Build history of the part. All positions in model axes, mm. Round coordinates to 2 decimals unless told otherwise and drop trailing zeros. Write each loop counter-clockwise with the first axis right and the second up, starting at its lowest first coordinate (ties: lowest second). Pieces come first, ordered by that corner, then holes. Notation, with made-up numbers: (48.5, -11) - (63.5, -11) arc R24 cw to (63.5, 16) - close; hole circle Ø9 at (51.25, -20). An arc over 180 degrees is marked (long way). One line per question, with ' | ' between items.
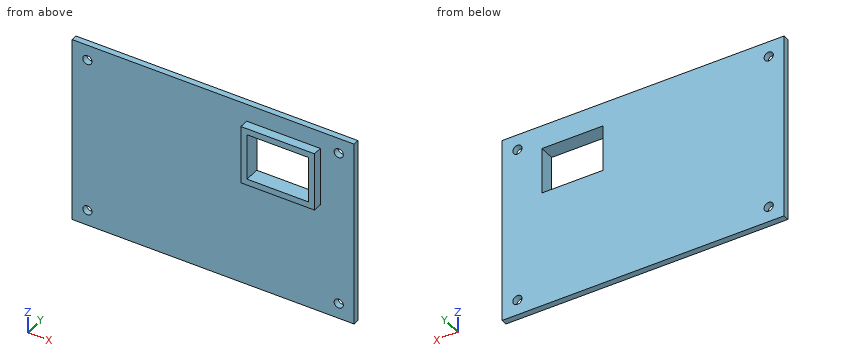
from build123d import *

# Parameters (mm, degrees)
SKETCH_1_W          = 92
SKETCH_1_H          = 60.74
EXTRUDE_1_DEPTH     = 2
SKETCH_2_R          = 1.5
CUT_EXTRUDE_1_DEPTH = 10
SKETCH_3_W          = 20
SKETCH_3_H          = 15
CUT_EXTRUDE_2_DEPTH = 10
SKETCH_4_W          = 24
SKETCH_4_H          = 19
SKETCH_4_W_2        = 20
SKETCH_4_H_2        = 15
EXTRUDE_2_DEPTH     = 3


with BuildPart() as part:
    # Эскиз1 → Бобышка-Вытянуть1 (new body)
    with BuildSketch(Plane(origin=(0, 0, 0), x_dir=(1, 0, 0), z_dir=(0, 1, 0))):
        Rectangle(SKETCH_1_W, SKETCH_1_H)
    extrude(amount=EXTRUDE_1_DEPTH)

    # Эскиз2 → Вырез-Вытянуть1 (cut)
    with BuildSketch(Plane(origin=(0, 2, 0), x_dir=(1, 0, 0), z_dir=(0, 1, 0))):
        with Locations((-41, 25.37)):
            Circle(SKETCH_2_R)
        with Locations((41, 25.37)):
            Circle(SKETCH_2_R)
        with Locations((41, -25.37)):
            Circle(SKETCH_2_R)
        with Locations((-41, -25.37)):
            Circle(SKETCH_2_R)
    extrude(amount=-CUT_EXTRUDE_1_DEPTH, mode=Mode.SUBTRACT)

    # Эскиз3 → Вырез-Вытянуть2 (cut)
    with BuildSketch(Plane(origin=(0, 2, 0), x_dir=(1, 0, 0), z_dir=(0, 1, 0))):
        with Locations((23, -15.185)):
            Rectangle(SKETCH_3_W, SKETCH_3_H)
    extrude(amount=-CUT_EXTRUDE_2_DEPTH, mode=Mode.SUBTRACT)

    # Эскиз4 → Бобышка-Вытянуть2 (add)
    with BuildSketch(Plane.XZ):
        with Locations((23, 15.185)):
            Rectangle(SKETCH_4_W, SKETCH_4_H)
        with Locations((23, 15.185)):
            Rectangle(SKETCH_4_W_2, SKETCH_4_H_2, mode=Mode.SUBTRACT)
    extrude(amount=EXTRUDE_2_DEPTH)


solid = part.part
Q1. Drill centre lines: L1, parallel to Z at x = 41, y = 1.2; L2, parallel to X at y = 1.25, z = -25.37; L3, parallel to X at y = 1.45, z = 22. Where is each one in solid material? Low to high. Write a range as from..to.
Found:
L1: -30.37..-26.87, -23.87..23.87, 26.87..30.37 | L2: -46..-42.5, -39.5..39.5, 42.5..46 | L3: -46..13, 33..46
Q2. Saw through at D-D, the plane y = -1.8. List the corners of the cut face in (x, z) (3 decimals), then the cut area to 3 significant figures.
Found:
outline: (11, 5.685) - (35, 5.685) - (35, 24.685) - (11, 24.685) - close; hole (13, 7.685) - (33, 7.685) - (33, 22.685) - (13, 22.685) - close | area: 156 mm^2
Q3. Saw through at B-B, the plane z = 11. List the corners of the cut face in (x, y), then the cut area to 3 significant figures.
Found:
outline: (-46, 0) - (11, 0) - (11, -3) - (13, -3) - (13, 2) - (-46, 2) - close; (33, -3) - (35, -3) - (35, 0) - (46, 0) - (46, 2) - (33, 2) - close | area: 156 mm^2
Q4. Saw through at A-A, the plane z = -25.37. List the corners of the cut face in (x, y).
Found:
outline: (-46, 0) - (-42.5, 0) - (-42.5, 2) - (-46, 2) - close; (-39.5, 0) - (39.5, 0) - (39.5, 2) - (-39.5, 2) - close; (42.5, 0) - (46, 0) - (46, 2) - (42.5, 2) - close
Q5. Drop flat-ended pins along their axis: pin 1 (0.9 mm diameter, centred on x = 27, y = -1.5, fed in from +Z) (3 decimals); pin 2 (4 mm diameter, centred on x = -41, z = -25.37, fed in from -Y); pin 3 (2.5 mm diameter, centred on y = -1.5, z = 19, fed in from -X); pin 4 (2.5 mm diameter, centred on x = 41, z = 25.37, fed in from -Y). Give the stop position or say it passes through.
Found:
pin 1: z = 24.685 | pin 2: y = 0 | pin 3: x = 11 | pin 4: through
Q6. Saw through at C-C, the plane x = 41. List the corners of the cut face in (y, z), then the cut area to 3 significant figures.
Found:
outline: (0, -30.37) - (2, -30.37) - (2, -26.87) - (0, -26.87) - close; (0, -23.87) - (2, -23.87) - (2, 23.87) - (0, 23.87) - close; (0, 26.87) - (2, 26.87) - (2, 30.37) - (0, 30.37) - close | area: 109 mm^2
